Geometry check sheet. Reference: the model listing, model coordinates, mm. A direction names the side the tool comes from. Round coordinates to 2 decimals unless told otherwise and drop trailing zeros. Write each loop counter-clockwise with the first axis right and the second up, starting at its lowest first coordinate (ties: lowest second). Pieces come first, ordered by that corner, then holes. Notation, with made-up numbers: M 20,36 L 73,36 A20 ccw 73,71 Z; hole C 79,71 d3. An arc over 180 degrees is marked long. One line per item, written item: value. Start each with the question number.
1. Depth check by flat-ended pin: P1, Ø1.5, axis at y = 18, z = 11, coming from the -X side; P2, Ø16, axis at x = -0.5, y = 8, coming from the -Z side (3 decimals); P3, Ø1.5, axis at y = 19.5, z = 12.5, coming from the +X side. Enter the tip coordinate at first touch or a pass-through.
2. Section check D-D (z = 16.5). Record the boundary of the cut face in (x, y), and give its area (3 significant figures).
3. Access from +Z, -Z, +X, -X, +Y, -Y to the whole of each face (thin tool, end or side, straight path). Record for faces 5 (the flat face through (23, 16.25, 10)), 6 (the flat face through (-23, 16.25, 10)), 7 (the flat face through (0, -5, 20)), 8 (the cylindrical face through (5.38, 17.28, 2.63)), 9 (the cylindrical face through (-2.17, -0.81, 17.37)).
4. Release check for a two-part mould opening along X. For faces 1 (the flat face through (-16.24, 22.01, 9.86)), 2 (the flat face through (2, 14, 14.675)), 3 (the flat face through (30, -1, 10)), 4 (the flat face through (-5, 7, 5.325)) record: pulls with the +X half, pulls with the -X half, needs draft (parallel to the pull), parting line crosses it, or undercut.
5. Section check A-A (z = 9.5). Record the boundary of the cut face in (x, y), and give its area (3 significant figures).
6. Scan lines: probe 1 along Y at (x, z) = (0, 8.25); probe 2 along Y at (x, z) = (0, 3.6); probe 3 along X at (y, z) = (8, 5.75). Record each from-to range of solid material in increasing order. Write a range as [from, to].
7. Section check C-C (y = 0). Record the boundary of the cut face in (x, z) (3 decimals).
8. Section check B-B (x = 0). Record the boundary of the cut face in (y, z) (3 decimals).
from build123d import *

# Parameters (mm, degrees)
SALIENTE_EXTRUIR1_DEPTH = 20
CROQUIS2_R              = 5
CORTAR_EXTRUIR1_DEPTH   = 21
CHAFL_N1_SIZE           = 1.5
CROQUIS3_R              = 10
CORTAR_EXTRUIR2_DEPTH   = 5.325
CROQUIS5_R              = 10
CORTAR_EXTRUIR3_DEPTH   = 5.325


with BuildPart() as part:
    # Croquis1 → Saliente-Extruir1 (new body)
    with BuildSketch(Plane.XY):
        Polygon((-30, 16.25), (-17, 16.25), (-17, 22.75), (17, 22.75), (17, 16.25), (30, 16.25), (30, -16.25), (-30, -16.25), align=None)
    extrude(amount=SALIENTE_EXTRUIR1_DEPTH)

    # Croquis2 → Cortar-Extruir1 (cut, through all)
    with BuildSketch(Plane.XY):
        with Locations((0, 8.95)):
            Circle(CROQUIS2_R)
    extrude(amount=CORTAR_EXTRUIR1_DEPTH, mode=Mode.SUBTRACT)

    # Chaflán1
    chafl_n1_edges = [part.edges().sort_by_distance(p)[0] for p in [
        (-30, 16.25, 10),
        (-17, 22.75, 10),
        (17, 22.75, 10),
        (30, 16.25, 10),
    ]]
    chamfer(chafl_n1_edges, length=CHAFL_N1_SIZE)

    # Croquis3 → Cortar-Extruir2 (cut)
    with BuildSketch(Plane.XY):
        with Locations((0, 8.851953405)):
            Circle(CROQUIS3_R)
    extrude(amount=CORTAR_EXTRUIR2_DEPTH, mode=Mode.SUBTRACT)

    # Croquis5 → Cortar-Extruir3 (cut)
    with BuildSketch(Plane.XY.offset(20)):
        with Locations((0, 8.95)):
            Circle(CROQUIS5_R)
    extrude(amount=-CORTAR_EXTRUIR3_DEPTH, mode=Mode.SUBTRACT)


solid = part.part
Result sheet:
1. P1: stops at x = -17
1. P2: stops at z = 5.325
1. P3: stops at x = 17
2. outline: M -30,-16.25 L 30,-16.25 L 30,14.75 L 28.5,16.25 L 17,16.25 L 17,21.25 L 15.5,22.75 L -15.5,22.75 L -17,21.25 L -17,16.25 L -28.5,16.25 L -30,14.75 Z; hole C 0,8.95 d20
2. area: 1,850 mm2
3. face 5: +Z, -Z, +X, +Y
3. face 6: +Z, -Z, -X, +Y
3. face 7: +Z, +X, -X, +Y, -Y
3. face 8: -Z
3. face 9: +Z
4. face 1: pulls with the -X half
4. face 2: undercut
4. face 3: pulls with the +X half
4. face 4: undercut
5. outline: M -30,-16.25 L 30,-16.25 L 30,14.75 L 28.5,16.25 L 17,16.25 L 17,21.25 L 15.5,22.75 L -15.5,22.75 L -17,21.25 L -17,16.25 L -28.5,16.25 L -30,14.75 Z; hole C 0,8.95 d10
5. area: 2,090 mm2
6. probe 1: y = [-16.25, 3.95], [13.95, 22.75]
6. probe 2: y = [-16.25, -1.15], [18.85, 22.75]
6. probe 3: x = [-30, -4.91], [4.91, 30]
7. outline: M -30,0 L -4.652,0 L -4.652,5.325 L 4.652,5.325 L 4.652,0 L 30,0 L 30,20 L 4.461,20 L 4.461,14.675 L -4.461,14.675 L -4.461,20 L -30,20 Z
8. outline: M -16.25,0 L -1.148,0 L -1.148,5.325 L 3.95,5.325 L 3.95,14.675 L -1.05,14.675 L -1.05,20 L -16.25,20 Z; M 13.95,5.325 L 18.852,5.325 L 18.852,0 L 22.75,0 L 22.75,20 L 18.95,20 L 18.95,14.675 L 13.95,14.675 Z
